from build123d import *

# Parameters (mm, degrees)
BOSS_EXTRUDE1_DEPTH   = 3.175
SKETCH2_R             = 9.525
CUT_EXTRUDE1_DEPTH    = 4.175
F_6_CLEARANCE_HOLE1_D = 4.3053
CUT_EXTRUDE2_DEPTH    = 4.175
F_6_CLEARANCE_HOLE2_D = 4.3053


with BuildPart() as part:
    # Sketch1 → Boss-Extrude1 (new body)
    with BuildSketch(Plane.XY):
        Polygon((0, 103.090949096), (0, 0), (62.688793586, 0), (62.688793586, 131), align=None)
    extrude(amount=-BOSS_EXTRUDE1_DEPTH)

    # Sketch2 → Cut-Extrude1 (cut, through all)
    with BuildSketch(Plane.XY):
        with Locations((32.143907641, 12.7)):
            Circle(SKETCH2_R)
        with Locations((47.270490427, 46.548006151)):
            Circle(SKETCH2_R)
        with Locations((47.270490427, 82.18542385)):
            Circle(SKETCH2_R)
        with Locations((20.373235059, 82.18542385)):
            Circle(SKETCH2_R)
        with Locations((20.373235059, 46.548006151)):
            Circle(SKETCH2_R)
    extrude(amount=-CUT_EXTRUDE1_DEPTH, mode=Mode.SUBTRACT)

    # #6 Clearance Hole1 (through all)
    with Locations(Plane.XY):
        with Locations((58.6105, 14.2875), (4.8895, 14.2875), (4.8895, 90.4875), (58.6105, 109.5375)):
            Hole(F_6_CLEARANCE_HOLE1_D / 2)

    # Sketch5 → Cut-Extrude2 (cut, through all)
    with BuildSketch(Plane.XY):
        with BuildLine():
            Line((0, 0), (11.24, 0))
            Line((11.24, 0), (11.24, 14.29))
            ThreePointArc((11.24, 14.29), (9.380128061, 18.780128061), (4.89, 20.64))
            Line((4.89, 20.64), (0, 20.64))
            Line((0, 20.64), (0, 0))
        make_face()
        with BuildLine():
            Line((51.448793586, 14.29), (51.448793586, 0))
            Line((51.448793586, 0), (62.688793586, 0))
            Line((62.688793586, 0), (62.688793586, 20.64))
            Line((62.688793586, 20.64), (57.798793586, 20.64))
            ThreePointArc((57.798793586, 20.64), (53.308665525, 18.780128061), (51.448793586, 14.29))
        make_face()
        with BuildLine():
            Line((0, 103.090949096), (0, 84.1375))
            Line((0, 84.1375), (4.8895, 84.1375))
            ThreePointArc((4.8895, 84.1375), (9.379628061, 85.997371939), (11.2395, 90.4875))
            Line((11.2395, 90.4875), (11.2395, 108.094774496))
            Line((11.2395, 108.094774496), (0, 103.090949096))
        make_face()
        with BuildLine():
            Line((62.688793586, 131), (62.688793586, 103.1875))
            Line((62.688793586, 103.1875), (58.6105, 103.1875))
            ThreePointArc((58.6105, 103.1875), (54.120371939, 105.047371939), (52.2605, 109.5375))
            Line((52.2605, 109.5375), (52.2605, 126.357323696))
            Line((52.2605, 126.357323696), (62.688793586, 131))
        make_face()
    extrude(amount=-CUT_EXTRUDE2_DEPTH, mode=Mode.SUBTRACT)

    # #6 Clearance Hole2 (through all)
    with Locations(Plane(origin=(31.750004441, 0, 3.175), x_dir=(1, 0, 0), z_dir=(0, 0, 1))):
        with Locations((1.676331213, 81.383391323), (-13.818696068, 17.771227958)):
            Hole(F_6_CLEARANCE_HOLE2_D / 2)


solid = part.part
Can you work these out from the model? Positions are in its coordinate system, mm. A direction names the side the tool comes from. Coordinates: 2 decimals unless noted, no trailing zeros. Order: outer loops, then holes, each group sorted by start corner. A loop starts at its lowest first (then second) coordinate and runs counter-clockwise, first axis right, second up. Notation, with made-up numbers: (40.25, -5.5) - (86.25, -5.5) arc R26 ccw to (86.25, 15.5) - close; hole circle Ø4 at (7, -12.75). An arc over 180 degrees is marked (long way). Answer as a JSON object with one key per item and string values. Group by question number.
Q1. Imagine slicing it at C-C (y = 48.5). Please give me the cut outline in (x, z) (3 decimals), and give its area (3 significant figures).
Q2. Imagine slicing it at B-B (x = 25.5). Please give me the cut outline in (y, z) (3 decimals), and give its area (3 significant figures).
Q3. We'd pull the mould along Y, two halves only. Please class faces 3 (the face through (60, 20.64, -2)), 4 (the face through (54.17, 105, -1.57)), 5 (the face through (13.353, 52.985, -1.565)), 6 (the face through (52.26, 118, -2)): +Y half, -Y half, draft (parallel to the pull), parting line (faces both ways), or undercut.
Q4. I need wall thicknesses on line 1 (Y direction, x = 40, z = -1.65); line 2 (X direction, y = 52, z = -1.25); line 3 (X direction, y = 80.5, z = -1.85). Which ranges of each line are inside material? Lowest first, please. Write a range as from..to.
Q5. On a 3-axis mill with a long thin cutter (end or side, diameter ignored), from which of +Z, -Z, +X, -X, +Y, -Y can I reach the whole of each face in a straight line? I mean faces 1 (the face through (62.689, 61, -2)), 2 (the face through (2, 20.64, -2)). Say none if no direction works.
Q6. Imagine slicing it at A-A (y = 12.7). Please give me the cut outline in (x, z) (3 decimals).
Q7. Imagine slicing it at D-D (x = 49). Please give me the cut outline in (y, z) (3 decimals).
Q8. Will these pins go through, and if not, where does the flat tip stop? P1, Ø11.5, axis at x = 20.37, y = 46.55, coming from the -Z side; P2, Ø1, axis at y = 100.5, z = -1.5, coming from the -X side; P3, Ø1, axis at y = 114.5, z = -2, coming from the +X side.
Determined:
{
 "1": {"outline": "(0, -3.175) - (11.05, -3.175) - (11.05, 0) - (0, 0) - close; (29.696, -3.175) - (37.948, -3.175) - (37.948, 0) - (29.696, 0) - close; (56.593, -3.175) - (62.689, -3.175) - (62.689, 0) - (56.593, 0) - close", "area": "80.6 mm2"},
 "2": {"outline": "(0, -3.175) - (5.875, -3.175) - (5.875, 0) - (0, 0) - close; (19.525, -3.175) - (38.52, -3.175) - (38.52, 0) - (19.525, 0) - close; (54.576, -3.175) - (74.158, -3.175) - (74.158, 0) - (54.576, 0) - close; (90.213, -3.175) - (114.444, -3.175) - (114.444, 0) - (90.213, 0) - close", "area": "218 mm2"},
 "3": {"face 3": "-Y half", "face 4": "+Y half", "face 5": "undercut", "face 6": "draft"},
 "4": {"line 1": "y = 0..7.31, 18.09..40.39, 52.7..76.03, 88.34..120.9", "line 2": "x = 0..12.56, 28.18..39.46, 55.08..62.69", "line 3": "x = 0..11, 29.75..31.46, 35.39..37.9, 56.65..62.69"},
 "5": {"face 1": "+Z, -Z, +X, +Y, -Y", "face 2": "+Z, -Z, -X, -Y"},
 "6": {"outline": "(11.24, -3.175) - (22.619, -3.175) - (22.619, 0) - (11.24, 0) - close; (41.669, -3.175) - (51.449, -3.175) - (51.449, 0) - (41.669, 0) - close"},
 "7": {"outline": "(0, -3.175) - (37.181, -3.175) - (37.181, 0) - (0, 0) - close; (55.915, -3.175) - (72.819, -3.175) - (72.819, 0) - (55.915, 0) - close; (91.552, -3.175) - (124.906, -3.175) - (124.906, 0) - (91.552, 0) - close"},
 "8": {"P1": "passes through", "P2": "stops at x = 11.24", "P3": "stops at x = 52.26"}
}
